Part print with two shaded views. Sizes in mm from the minimum x, y, z corner. Round coordinates to 2 decimals unless told otherwise and drop trailing zeros. Loops run counter-clockwise (first coordinate to the right, second up) from the corner with the lowest first, then second, coordinate; pieces in that order, holes last. Notation, with made-up numbers: (47.5, 17.25) -> (62.5, 17.25) arc R27 cw to (62.5, 36.25) -> close; hole circle Ø9 at (46, 37.25). An arc over 180 degrees is marked (long way). Answer as a JSON object with one key per item and string values. Group by question number.
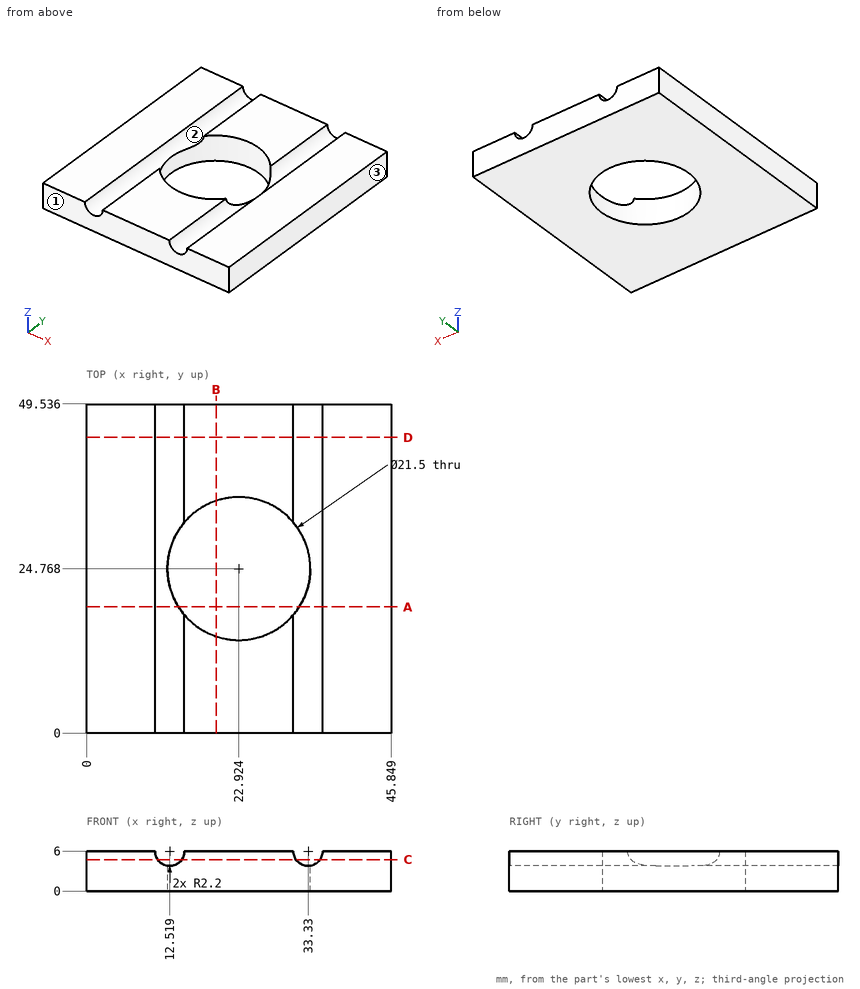
Item 1: Drill centre lines: line 1 (X direction, y = 6, z = 4.5); line 2 (X direction, y = 27, z = 5.75) (1 decimal); line 3 (Y direction, x = 23, z = 5.25) (1 decimal). Where is each one in solid material? Low to high.
Item 2: Band-saw the part on C-C, the plane z = 4.75. Count the separate pieces of the cut face and the enclosed holes in it, plus the area to 3 significant figures.
Item 3: Band-saw the part on A-A, the plane y = 19. List the corners of the cut face in (x, z), plus the area to 3 significant figures.
Item 4: Two-plate mould, pull along X, no slides. Class the marked faces 1, 2 and 3: pulls with the +X half, pulls with the -X half, needs draft (parallel to the pull), parting line crosses it, or undercut.
Item 5: Drop a flat-ended pin along its axis: pin 1 Ø13 at (x, y) = (22.92, 24.77) entering from +Z. Give the stop position or say it passes through.
Item 6: Band-saw the part on D-D, the plane y = 44.5. List the corners of the cut face in (x, z), plus the area to 3 significant figures.
Item 7: Band-saw the part on B-B, the plane x = 19.5. List the corners of the cut face in (y, z) (1 decimal), plus the area to 3 significant figures.
Entries:
{
 "1": {"line 1": "0 to 10.91, 14.13 to 31.72, 34.94 to 45.85", "line 2": "0 to 10.3, 35.5 to 45.8", "line 3": "0 to 14, 35.5 to 49.5"},
 "2": {"separate pieces": "4", "enclosed holes": "0", "area": "1,590 mm²"},
 "3": {"outline": "(0, 0) -> (13.85, 0) -> (13.85, 4.25) arc R2.2 cw to (10.32, 6) -> (0, 6) -> close; (32, 0) -> (45.85, 0) -> (45.85, 6) -> (35.53, 6) arc R2.2 cw to (32, 4.25) -> close", "area": "153 mm²"},
 "4": {"face 1": "needs draft", "face 2": "undercut", "face 3": "pulls with the +X half"},
 "5": {"pin 1": "through"},
 "6": {"outline": "(0, 0) -> (45.85, 0) -> (45.85, 6) -> (35.53, 6) arc R2.2 cw to (31.13, 6) -> (14.72, 6) arc R2.2 cw to (10.32, 6) -> (0, 6) -> close", "area": "260 mm²"},
 "7": {"outline": "(0, 0) -> (14.6, 0) -> (14.6, 6) -> (0, 6) -> close; (35, 0) -> (49.5, 0) -> (49.5, 6) -> (35, 6) -> close", "area": "175 mm²"}
}
